from build123d import *

# Parameters (mm, degrees)
SKETCH_1_R          = 15.75
SKETCH_1_R_2        = 1.6
EXTRUDE_1_DEPTH     = 3
EXTRUDE_2_DEPTH     = 3
SKETCH_3_W          = 20
SKETCH_3_H          = 31.5
EXTRUDE_3_DEPTH     = 5
SKETCH_4_R          = 1.6
CUT_EXTRUDE_1_DEPTH = 10


with BuildPart() as part:
    # 草图1 → 凸台-拉伸1 (new body)
    with BuildSketch(Plane(origin=(0, 0, 0), x_dir=(1, 0, 0), z_dir=(0, 1, 0))):
        Circle(SKETCH_1_R)
        with Locations((0, 8)):
            Circle(SKETCH_1_R_2, mode=Mode.SUBTRACT)
        with Locations((8, 0)):
            Circle(SKETCH_1_R_2, mode=Mode.SUBTRACT)
        with Locations((0, -8)):
            Circle(SKETCH_1_R_2, mode=Mode.SUBTRACT)
        with Locations((-8, 0)):
            Circle(SKETCH_1_R_2, mode=Mode.SUBTRACT)
    extrude(amount=EXTRUDE_1_DEPTH)

    # 草图2 → 凸台-拉伸2 (add)
    with BuildSketch(Plane.XZ):
        with BuildLine():
            Line((0, 15.75), (55, 15.75))
            Line((55, 15.75), (55, -15.75))
            Line((55, -15.75), (0, -15.75))
            ThreePointArc((0, -15.75), (15.75, 0), (0, 15.75))
        make_face()
    extrude(amount=-EXTRUDE_2_DEPTH)

    # 草图3 → 凸台-拉伸3 (add)
    with BuildSketch(Plane.XZ):
        with Locations((45, 0)):
            Rectangle(SKETCH_3_W, SKETCH_3_H)
    extrude(amount=-EXTRUDE_3_DEPTH)

    # 草图4 → 切除-拉伸1 (cut)
    with BuildSketch(Plane(origin=(0, 5, 0), x_dir=(1, 0, 0), z_dir=(0, 1, 0))):
        with Locations((45, 4.5)):
            Circle(SKETCH_4_R)
        with Locations((45, -4.5)):
            Circle(SKETCH_4_R)
    extrude(amount=-CUT_EXTRUDE_1_DEPTH, mode=Mode.SUBTRACT)


solid = part.part
The model under review builds one solid part; all positions refer to its coordinate system, in mm. A direction names the side the tool comes from. Round coordinates to 2 decimals unless told otherwise and drop trailing zeros. Write each loop counter-clockwise with the first axis right and the second up, starting at its lowest first coordinate (ties: lowest second). Pieces come first, ordered by that corner, then holes. Notation, with made-up numbers: (11, 37.5) -> (33, 37.5) arc R26 ccw to (33, 52.5) -> close; hole circle Ø1 at (-18, 70.25). An arc over 180 degrees is marked (long way). Answer as a JSON object with one key per item and string values.
1. Clearance check with flat-ended pins moving along their axes: pin 1 (0.6 mm diameter, centred on y = 4, z = -2.5, fed in from -X); pin 2 (5 mm diameter, centred on x = -8, z = 0, fed in from +Y); pin 3 (2 mm diameter, centred on x = -4, y = 2.5, fed in from +Z). State where each tip first meets the part, or that it passes through.
Results found:
{"pin 1": "stops at x = 35", "pin 2": "stops at y = 3", "pin 3": "stops at z = 15.46"}
2. We need section C-C on x = 45. State the section outline as (y, z) points.
Results found:
{"outline": "(0, -15.75) -> (5, -15.75) -> (5, -6.1) -> (0, -6.1) -> close; (0, -2.9) -> (5, -2.9) -> (5, 2.9) -> (0, 2.9) -> close; (0, 6.1) -> (5, 6.1) -> (5, 15.75) -> (0, 15.75) -> close"}
3. We need section B-B on y = 1.3. State the section outline as (x, z) points.
Results found:
{"outline": "(0, -15.75) -> (55, -15.75) -> (55, 15.75) -> (0, 15.75) arc R15.75 ccw to start; hole circle Ø3.2 at (-8, 0); hole circle Ø3.2 at (0, -8); hole circle Ø3.2 at (0, 8); hole circle Ø3.2 at (8, 0); hole circle Ø3.2 at (45, -4.5); hole circle Ø3.2 at (45, 4.5)"}
4. We need section A-A on x = 8. State the section outline as (y, z) points, and give its area (3 significant figures).
Results found:
{"outline": "(0, -15.75) -> (3, -15.75) -> (3, -1.6) -> (0, -1.6) -> close; (0, 1.6) -> (3, 1.6) -> (3, 15.75) -> (0, 15.75) -> close", "area": "84.9 mm^2"}
5. To check wall thickness, follow line 1 along Z through (x, y) = (45, 2.3); line 2 along X through (y, z) = (2.1, 0); line 3 along Z through (x, y) = (8, 2.3). State the ranges of each line that lie inside material, in increasing order.
Results found:
{"line 1": "z = -15.75 to -6.1, -2.9 to 2.9, 6.1 to 15.75", "line 2": "x = -15.75 to -9.6, -6.4 to 6.4, 9.6 to 55", "line 3": "z = -15.75 to -1.6, 1.6 to 15.75"}
6. We need section D-D on z = -4.5. State the section outline as (x, y) points, and give its area (3 significant figures).
Results found:
{"outline": "(-15.09, 0) -> (43.4, 0) -> (43.4, 5) -> (35, 5) -> (35, 3) -> (-15.09, 3) -> close; (46.6, 0) -> (55, 0) -> (55, 5) -> (46.6, 5) -> close", "area": "234 mm^2"}
7. Machinability: for faces 1 (the face through (10, 3, 0)), 2 (the face through (45.74, 2.54, 5.92)), which of the approach directions +Z, -Z, +X, -X, +Y, -Y give a long, thin tool a straight path to every point of the face, cutting with its end or side? Answer none if there is none.
Results found:
{"face 1": "+Z, -Z, -X, +Y", "face 2": "+Y, -Y"}
8. The part is to be moulded in two halves that separate along X. For faces 3 (the face through (-15.746, 1.479, -0.346)), 4 (the face through (6.4, 1.48, -0.07)), 5 (the face through (-9.6, 1.48, -0.07)), 6 (the face through (34, 2, -15.75)), say which applies: pulls with the +X half, pulls with the -X half, needs draft (parallel to the pull), parting line crosses it, or undercut.
Results found:
{"face 3": "pulls with the -X half", "face 4": "undercut", "face 5": "undercut", "face 6": "needs draft"}
